```python
from build123d import *

# Parameters (mm, degrees)
SKETCH1_R           = 49.375
SKETCH1_R_2         = 39.375
BOSS_EXTRUDE1_DEPTH = 13
CUT_EXTRUDE1_REACH  = 73.027
SKETCH2_R           = 1.5
CIRPATTERN1_COUNT   = 6


with BuildPart() as part:
    # Sketch1 → Boss-Extrude1 (new body)
    with BuildSketch(Plane(origin=(0, 0, 0), x_dir=(1, 0, 0), z_dir=(0, 1, 0))):
        with Locations(Location((0, 0, 0), (0, 0, 90))):
            Circle(SKETCH1_R)
        with Locations(Location((0, 0, 0), (0, 0, 90))):
            Circle(SKETCH1_R_2, mode=Mode.SUBTRACT)
    extrude(amount=BOSS_EXTRUDE1_DEPTH)

    # Sketch2 → Cut-Extrude1 (cut, up to next)
    with BuildSketch(Plane(origin=(0, 13, 0), x_dir=(1, 0, 0), z_dir=(0, 1, 0)), mode=Mode.PRIVATE) as cut_extrude1_sk1:
        with Locations(Location((-7.5, -44.370598373, 0), (0, 0, 270))):
            Circle(SKETCH2_R)
    cut_extrude1_tool1 = extrude(cut_extrude1_sk1.sketch, amount=-CUT_EXTRUDE1_REACH, mode=Mode.PRIVATE) & part.part
    # Sketch2 → Cut-Extrude1 (cut, up to next)
    with BuildSketch(Plane(origin=(0, 13, 0), x_dir=(1, 0, 0), z_dir=(0, 1, 0)), mode=Mode.PRIVATE) as cut_extrude1_sk2:
        with Locations(Location((7.5, -44.370598373, 0), (0, 0, 270))):
            Circle(SKETCH2_R)
    cut_extrude1_tool2 = extrude(cut_extrude1_sk2.sketch, amount=-CUT_EXTRUDE1_REACH, mode=Mode.PRIVATE) & part.part
    cut_extrude1_1 = cut_extrude1_tool1.solids().sort_by_distance((-7.5, 13, 44.370598))[0]
    add(cut_extrude1_1, mode=Mode.SUBTRACT)
    cut_extrude1_2 = cut_extrude1_tool2.solids().sort_by_distance((7.5, 13, 44.370598))[0]
    add(cut_extrude1_2, mode=Mode.SUBTRACT)
    cut_extrude1 = cut_extrude1_1 + cut_extrude1_2  # Cut-Extrude1 as one shape, for the pattern or mirror that repeats it

    # CirPattern1: Cut-Extrude1 ×6 about axis
    cirpattern1_axis = Axis((0, 0, 0), (0, 1, 0))
    for i in range(1, CIRPATTERN1_COUNT):
        add(cut_extrude1.rotate(cirpattern1_axis, i * 360 / CIRPATTERN1_COUNT), mode=Mode.SUBTRACT)


solid = part.part
```
Verification items for the finished model (mm, model axes). Give positions to 0.01 mm unless a question says otherwise; leave off trailing zeros. Loops run counter-clockwise (first coordinate to the right, second up) from the corner with the lowest first, then second, coordinate; pieces in that order, holes last. Notation, with made-up numbers: M -17.5,39.5 L 11.5,39.5 A20 ccw 11.5,54.5 Z; hole C 79,-32.75 d4. An arc over 180 degrees is marked long. One line per question, with ' | ' between items.
Item 1: Depth check by flat-ended pin: P1, Ø4, axis at x = -25.5, y = 4.5, coming from the +Z side; P2, Ø6, axis at y = 3, z = 28.5, coming from the -X side; P3, Ø5, axis at y = 2.5, z = -8.5, coming from the +X side. Enter the tip coordinate at first touch or a pass-through.
Completed:
P1: stops at z = 43.42 | P2: stops at x = -42.28 | P3: stops at x = 49.01
Item 2: Section check B-B, the plane x = 0. Record the cut outline in (y, z) (3 decimals), plus the area to 3 significant figures.
Completed:
outline: M 0,-49.375 L 13,-49.375 L 13,-39.375 L 0,-39.375 Z; M 0,39.375 L 13,39.375 L 13,49.375 L 0,49.375 Z | area: 260 mm^2
Item 3: Thickness scan on line 1 (X direction, y = 5, z = 0) (3 decimals); line 2 (X direction, y = 3, z = -29); line 3 (X direction, y = 8, z = 45). Record the ranges inside material, lowest first. Write a range as [from, to].
Completed:
line 1: x = [-49.375, -39.375], [39.375, 49.375] | line 2: x = [-39.96, -36.14], [-33.21, -26.63], [26.63, 33.21], [36.14, 39.96] | line 3: x = [-20.32, -8.86], [-6.14, 6.14], [8.86, 20.32]
Item 4: Draft check along X on faces 1 (the face through (-14.831, 6.409, -47.095)), 2 (the face through (38.439, 6.409, 8.536)), 3 (the face through (-37, 13, -14)). Enter one of: +X half, -X half, draft (parallel to the pull), parting line (faces both ways), or undercut.
Completed:
face 1: parting line | face 2: undercut | face 3: draft
Item 5: Section check A-A, the plane z = 0. Record the cut outline in (x, y) (3 decimals), plus the area to 3 significant figures.
Completed:
outline: M -49.375,0 L -39.375,0 L -39.375,13 L -49.375,13 Z; M 39.375,0 L 49.375,0 L 49.375,13 L 39.375,13 Z | area: 260 mm^2
Item 6: Section check C-C, the plane y = 2.25. State how many separate pieces and enclosed holes the cut face has, plus the area to 3 significant figures.
Completed:
separate pieces: 1 | enclosed holes: 13 | area: 2,700 mm^2
